Part model, mm, in its own coordinate system. A direction names the side the tool comes from. Coordinates: 2 decimals unless noted, no trailing zeros. Loops run counter-clockwise (first coordinate to the right, second up) from the corner with the lowest first, then second, coordinate; pieces in that order, holes last. Notation, with made-up numbers: M 77.25,-13.75 L 83.25,-13.75 A14 ccw 83.25,6.25 Z; hole C 40.25,-2 d7. An arc over 180 degrees is marked long. Use a Markdown table: item, result. Add a question column.
1) Band-saw the part on A-A (x = 6). State how many separate pieces and enclosed holes the cut face has, plus the area to 3 significant figures.
2) Wall check: probe 1 along Y at (x, z) = (4.25, 7.2); probe 2 along X at (y, z) = (5, 68); probe 3 along X at (y, z) = (3, 25). Give the ranges that are in metal, low to high. Write a range as from..to.
3) Band-saw the part on B-B (z = 80.2). List the corners of the cut face in (x, y), plus the area to 3 significant figures.
4) Pin check, flat tips, straight feed: pin 1 Ø3 at (y, z) = (2, 24) entering from +X; pin 2 Ø2 at (x, z) = (0.5, 18.5) entering from +Y; pin 3 Ø3 at (x, z) = (1.5, 51.5) entering from +Y. Stop position of each tip, or through.
5) Pull direction Y, two halves, no side cores. Call faces 4 (the cylindrical face through (3.4, 2.5, 40.1)), 5 (the flat face through (2, 4.8, 41)), 6 (the flat face through (5, 3, 46.3)): released by +Y, released by -Y, zero draft, split by the parting line, or undercut.
6) Tool access for faces 1 (the flat face through (1, 3, 46.3)), 2 (the flat face through (6.8, 3, 78)), 3 (the flat face through (5, 3, 36.7)): list every direction of +Z, -Z, +X, -X, +Y, -Y with a clear straight run to the whole face (end or side of a thin tool).
7) Band-saw the part on C-C (z = 59). List the corners of the cut face in (x, y).
from build123d import *

# Parameters (mm, degrees)
BOSS_EXTRUDE1_DEPTH         = 9.8
BOSS_EXTRUDE2_DEPTH         = 26.9
BOSS_EXTRUDE3_DEPTH         = 9.6
BOSS_EXTRUDE4_DEPTH         = 26.9
BOSS_EXTRUDE5_DEPTH         = 9.8
TAP_DRILL_FOR_M2X0_4_TAP1_D = 1.6


with BuildPart() as part:
    # Sketch2 → Boss-Extrude1 (new body)
    with BuildSketch(Plane.XY):
        Polygon((0, 0), (6.8, 0), (6.8, 6.2), (3.7, 6.2), (2.5, 5), (2.5, 4.8), (0, 4.8), align=None)
    extrude(amount=BOSS_EXTRUDE1_DEPTH)

    # Sketch3 → Boss-Extrude2 (add)
    with BuildSketch(Plane.XY.offset(9.8)):
        Polygon((0, 0), (0, 1.6), (1.9, 1.6), (1.9, 4.8), (2.5, 4.8), (2.5, 5), (3.7, 6.2), (4, 6.2), (4, 0), align=None)
    extrude(amount=BOSS_EXTRUDE2_DEPTH)

    # Sketch6 → Boss-Extrude3 (add)
    with BuildSketch(Plane.XY.offset(36.7)):
        Polygon((0, 0), (6.8, 0), (6.8, 6.2), (3.7, 6.2), (2.5, 5), (2.5, 4.8), (0, 4.8), align=None)
    extrude(amount=BOSS_EXTRUDE3_DEPTH)

    # Sketch7 → Boss-Extrude4 (add)
    with BuildSketch(Plane.XY.offset(46.3)):
        Polygon((0, 0), (0, 1.6), (1.9, 1.6), (1.9, 4.8), (2.5, 4.8), (2.5, 5), (3.7, 6.2), (4, 6.2), (4, 0), align=None)
    extrude(amount=BOSS_EXTRUDE4_DEPTH)

    # Sketch8 → Boss-Extrude5 (add)
    with BuildSketch(Plane.XY.offset(73.2)):
        Polygon((0, 0), (6.8, 0), (6.8, 6.2), (3.7, 6.2), (2.5, 5), (2.5, 4.8), (0, 4.8), align=None)
    extrude(amount=BOSS_EXTRUDE5_DEPTH)

    # Tap Drill for M2x0.4 Tap1 (through all)
    with Locations(Plane.ZY):
        with Locations((7.2, 2.5), (2.8, 2.5), (39.3, 2.5), (43.7, 2.5), (75.8, 2.5), (80.2, 2.5)):
            Hole(TAP_DRILL_FOR_M2X0_4_TAP1_D / 2)


solid = part.part
Entries:
| question | item | result |
|---|---|---|
| 1 | separate pieces | 3 |
| 1 | enclosed holes | 6 |
| 1 | area | 169 mm2 |
| 2 | probe 1 | 0..1.7, 3.3..6.2 |
| 2 | probe 2 | 2.5..4 |
| 2 | probe 3 | 1.9..4 |
| 3 | outline | M 0,0 L 6.8,0 L 6.8,1.7 L 0,1.7 Z; M 0,3.3 L 6.8,3.3 L 6.8,6.2 L 3.7,6.2 L 2.5,5 L 2.5,4.8 L 0,4.8 Z |
| 3 | area | 27.1 mm2 |
| 4 | pin 1 | x = 4 |
| 4 | pin 2 | y = 1.6 |
| 4 | pin 3 | y = 5.5 |
| 5 | face 4 | undercut |
| 5 | face 5 | released by +Y |
| 5 | face 6 | zero draft |
| 6 | face 1 | -X, +Y |
| 6 | face 2 | +Z, -Z, +X, +Y, -Y |
| 6 | face 3 | +X, +Y, -Y |
| 7 | outline | M 0,0 L 4,0 L 4,6.2 L 3.7,6.2 L 2.5,5 L 2.5,4.8 L 1.9,4.8 L 1.9,1.6 L 0,1.6 Z |
